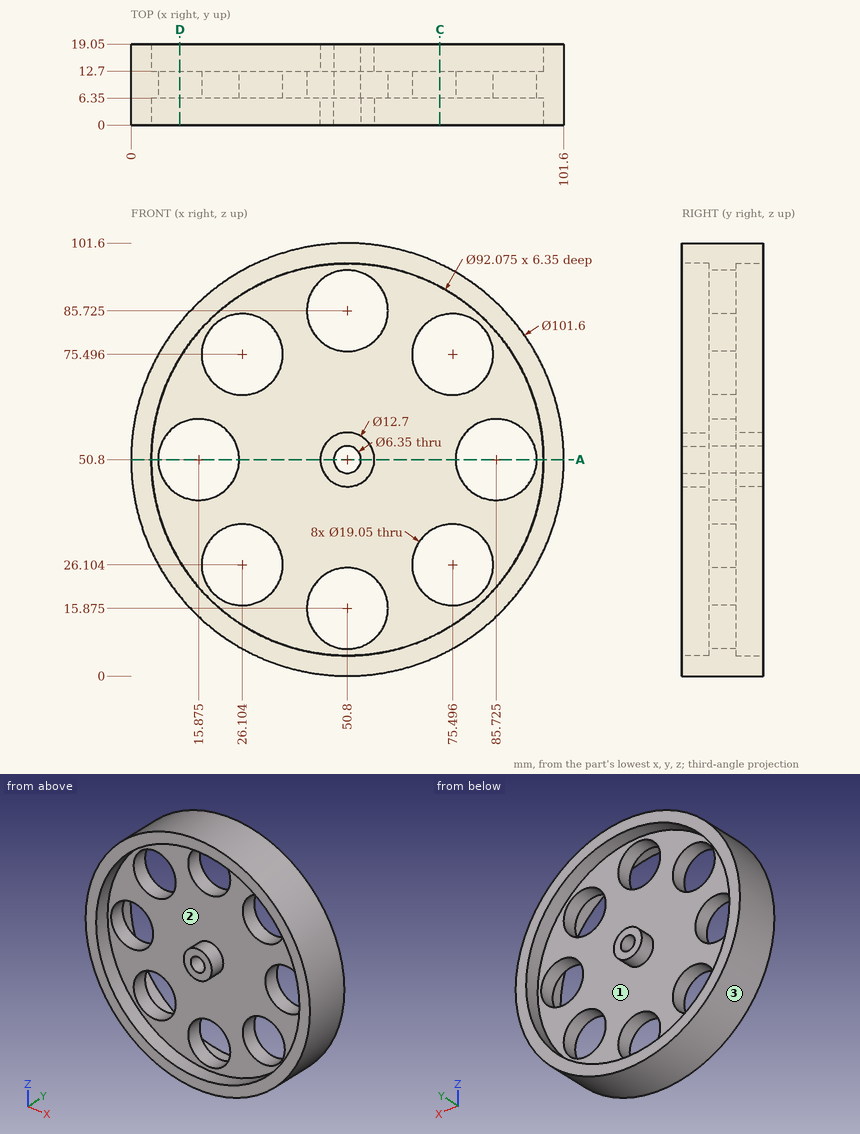
Answer from the drawing. Dimensions are ordinates in mm from the lowest x, y and z of the part. Round coordinates to 2 decimals unless told otherwise and drop trailing zeros. Order: outer loops, then holes, each group sorted by start corner. A loop starts at its lowest first (then second) coordinate and runs counter-clockwise, first axis right, second up.
1) The part is cut by section C-C on x = 72.5. Write down the section's boundary in (y, z), plus the area to 3 significant figures.
2) The part is cut by section A-A on z = 50.8. Give the number of separate pieces and of enclosed holes in the cut face.
3) The mould has two halves that part along Z. Classify the marked faces 1, 2 and 3: released by +Z, released by -Z, zero draft, split by the parting line, or undercut.
4) Flat-ended cylindrical pins translate along their axes: pin 1 (22 mm diameter, centred on x = 26.1, z = 26.1, fed in from +Y); pin 2 (1.5 mm diameter, centred on x = 67.5, z = 74.5, fed in from +Y); pin 3 (5 mm diameter, centred on y = 13.5, z = 79, fed in from +X); pin 4 (8.5 mm diameter, centred on x = 50.8, z = 50.8, fed in from +Y). Find the tip coordinate at first contact, or state that the pin passes through.
5) The part is cut by section D-D on x = 11.5. Write down the section's boundary in (y, z).
6) Straight lines are drawn through the part: L1, parallel to X at y = 11.25, z = 34 (1 decimal); L2, parallel to Z at x = 53, y = 14.5 (1 decimal); L3, parallel to X at y = 2, z = 46.5 (1 decimal). For each, find the intervals that lie inside material, in ascending order.
Resolved:
1. outline: (0, 4.87) - (19.05, 4.87) - (19.05, 10.2) - (12.7, 10.2) - (12.7, 17.06) - (6.35, 17.06) - (6.35, 10.2) - (0, 10.2) - close; (0, 91.4) - (6.35, 91.4) - (6.35, 84.54) - (12.7, 84.54) - (12.7, 91.4) - (19.05, 91.4) - (19.05, 96.73) - (0, 96.73) - close; (6.35, 35.15) - (12.7, 35.15) - (12.7, 66.45) - (6.35, 66.45) - close
1. area: 489 mm2
2. separate pieces: 4
2. enclosed holes: 0
3. face 1: undercut
3. face 2: undercut
3. face 3: split by the parting line
4. pin 1: stops at y = 12.7
4. pin 2: passes through
4. pin 3: stops at x = 94.62
4. pin 4: stops at y = 19.05
5. outline: (0, 18.61) - (19.05, 18.61) - (19.05, 26.82) - (12.7, 26.82) - (12.7, 42.34) - (6.35, 42.34) - (6.35, 26.82) - (0, 26.82) - close; (0, 74.78) - (6.35, 74.78) - (6.35, 59.26) - (12.7, 59.26) - (12.7, 74.78) - (19.05, 74.78) - (19.05, 82.99) - (0, 82.99) - close
6. L1: x = 2.9 to 20.8, 31.4 to 70.2, 80.8 to 98.7
6. L2: z = 0 to 4.8, 44.8 to 48.5, 53.1 to 56.8, 96.8 to 101.6
6. L3: x = 0.2 to 5, 46.1 to 55.5, 96.6 to 101.4
